Part model, mm, in its own coordinate system. Give positions to 0.01 mm unless a question says otherwise; leave off trailing zeros. Write each loop counter-clockwise with the first axis right and the second up, starting at its lowest first coordinate (ties: lowest second). Pieces come first, ordered by that corner, then holes. Notation, with made-up numbers: M 84,64 L 106,64 A31 cw 106,102 Z; hole C 29.25,24 d11. An arc over 180 degrees is marked long. Write item = value, one per line. Start each with the question number.
from build123d import *

# Parameters (mm, degrees)
SZKIC1_R                    = 22
SZKIC1_R_2                  = 12.5
DODANIE_WYCI_GNI_CIE1_DEPTH = 4
SFAZOWANIE1_SIZE            = 0.5


with BuildPart() as part:
    # Szkic1 → Dodanie-wyciągnięcie1 (new body)
    with BuildSketch(Plane.XY):
        Circle(SZKIC1_R)
        Circle(SZKIC1_R_2, mode=Mode.SUBTRACT)
    extrude(amount=DODANIE_WYCI_GNI_CIE1_DEPTH)

    # Sfazowanie1
    sfazowanie1_edges = [part.edges().sort_by_distance(p)[0] for p in [
        (-22, 0, 0),
        (-22, 0, 4),
        (-12.5, 0, 0),
        (-12.5, 0, 4),
    ]]
    chamfer(sfazowanie1_edges, length=SFAZOWANIE1_SIZE)


solid = part.part
Q1. Slice it at C-C (z = 2.15). Give the cut face in (x, y), and give its area (3 significant figures).
Q2. Two-plate mould, pull along X, no slides. Class faces 1 (the face through (11.923, 3.755, 1.979)), 2 (the face through (-4.769, -21.477, 1.979)), 3 (the face through (9.3, -9.3, 0)): +X half, -X half, draft (parallel to the pull), parting line (faces both ways), or undercut.
Q3. Probe line 1 along Y through (x, z) = (0, 2.05); line 2 along Y through (x, z) = (-7.5, 1.9); line 3 along X through (y, z) = (1.5, 3.7). List the from-to ranges inside material, lowest first.
Q4. Drop flat-ended pins along their axis: P1, Ø22.5, axis at x = 0, y = 0, coming from the +Z side; P2, Ø1.5, axis at y = -13, z = 2.5, coming from the +X side; P3, Ø1.5, axis at x = 16.5, z = 3.5, coming from the -Y side; P4, Ø2, axis at y = 7, z = 3.5, coming from the +X side. Give the stop position or say it passes through.
Q5. Slice it at A-A (x = 0). Give the cut face in (y, z).
Working result:
q1.outline = C 0,0 d44; hole C 0,0 d25
q1.area = 1,030 mm2
q2.face_1 = undercut
q2.face_2 = parting line
q2.face_3 = draft
q3.line_1 = -22 to -12.5, 12.5 to 22
q3.line_2 = -20.68 to -10, 10 to 20.68
q3.line_3 = -21.75 to -12.61, 12.61 to 21.75
q4.P1 = through
q4.P2 = 18.27
q4.P3 = -15.36
q4.P4 = 21.17
q5.outline = M -22,0.5 L -21.5,0 L -13,0 L -12.5,0.5 L -12.5,3.5 L -13,4 L -21.5,4 L -22,3.5 Z; M 12.5,0.5 L 13,0 L 21.5,0 L 22,0.5 L 22,3.5 L 21.5,4 L 13,4 L 12.5,3.5 Z
